```python
from build123d import *

# Parameters (mm, degrees)
CROQUIS1_W              = 77.5
CROQUIS1_H              = 52.5
SALIENTE_EXTRUIR1_DEPTH = 30
VACIADO1_T              = -2
CROQUIS2_R              = 1.75
CORTAR_EXTRUIR1_DEPTH   = 30


with BuildPart() as part:
    # Croquis1 → Saliente-Extruir1 (new body)
    with BuildSketch(Plane(origin=(0, 0, 0), x_dir=(1, 0, 0), z_dir=(0, 1, 0))):
        Rectangle(CROQUIS1_W, CROQUIS1_H)
    extrude(amount=SALIENTE_EXTRUIR1_DEPTH)

    # Vaciado1
    vaciado1_openings = [part.faces().sort_by_distance(p)[0] for p in [
        (0, 30, 0),
    ]]
    offset(amount=VACIADO1_T, openings=vaciado1_openings, kind=Kind.INTERSECTION)

    # Croquis2 → Cortar-Extruir1 (cut, symmetric)
    with BuildSketch(Plane(origin=(0, 2, 0), x_dir=(1, 0, 0), z_dir=(0, 1, 0))):
        with Locations(Location((-36.25, 23.75, 0), (0, 0, 270))):
            Circle(CROQUIS2_R)
        with Locations(Location((36.25, 23.75, 0), (0, 0, 270))):
            Circle(CROQUIS2_R)
        with Locations(Location((36.25, -23.75, 0), (0, 0, 270))):
            Circle(CROQUIS2_R)
        with Locations(Location((-36.25, -23.75, 0), (0, 0, 270))):
            Circle(CROQUIS2_R)
    extrude(amount=CORTAR_EXTRUIR1_DEPTH, both=True, mode=Mode.SUBTRACT)


solid = part.part
```
Design review of the part built by this model. Coordinates are the model's own, in mm. A direction names the side the tool comes from. Coordinates: 2 decimals unless noted, no trailing zeros. Order: outer loops, then holes, each group sorted by start corner. A loop starts at its lowest first (then second) coordinate and runs counter-clockwise, first axis right, second up. Notation, with made-up numbers: M 42,78 L 97,78 A24 ccw 97,114 Z; hole C 12,56 d9. An arc over 180 degrees is marked long. Answer as a JSON object with one key per item and string values. Group by question number.
1) Wall thickness on L1, parallel to Z at x = 36.25, y = 0.5; L2, parallel to X at y = 0.85, z = -23.75; L3, parallel to X at y = 12.5, z = -23.75: over which ranges is each line inside the solid? List them lowest first.
2) Add section A-A, the plane y = 21.5. Write out the cut boundary in (x, z).
3) Mouldability with a two-part tool opening along Z and no side actions: class faces 1 (the flat face through (-1, 15, 26.25)), 2 (the flat face through (-1, 0, 0)), 3 (the flat face through (0, 16, 24.25)) as pulls with the +Z half, pulls with the -Z half, needs draft (parallel to the pull), parting line crosses it, or undercut.
4) Add section B-B, the plane z = 4. Write out the cut boundary in (x, y), then the cut area to 3 significant figures.
5) For pin 1 (1.5 mm diameter, centred on x = -17.5, z = 15.5, fed in from +Y), flat-tipped, find the tip position at first contact; note if it passes through.
6) Add section C-C, the plane x = 16. Write out the cut boundary in (y, z).
7) Tool access review of faces 4 (the flat face through (-1, 2, 0)), 5 (the flat face through (-1, 15, -26.25)): name each direction out of +Z, -Z, +X, -X, +Y, -Y from which nothing blocks a thin tool from reaching the whole face with its end or side.
Computed values:
{
 "1": {"L1": "z = -26.25 to -25.5, -22 to 22, 25.5 to 26.25", "L2": "x = -38.75 to -38, -34.5 to 34.5, 38 to 38.75", "L3": "x = -38.75 to -38, 38 to 38.75"},
 "2": {"outline": "M -38.75,-26.25 L 38.75,-26.25 L 38.75,26.25 L -38.75,26.25 Z; hole M -36.75,-22.07 A1.75 ccw long -34.57,-24.25 L 34.57,-24.25 A1.75 ccw long 36.75,-22.07 L 36.75,22.07 A1.75 ccw long 34.57,24.25 L -34.57,24.25 A1.75 ccw long -36.75,22.07 Z"},
 "3": {"face 1": "pulls with the +Z half", "face 2": "needs draft", "face 3": "undercut"},
 "4": {"outline": "M -38.75,0 L 38.75,0 L 38.75,30 L 36.75,30 L 36.75,2 L -36.75,2 L -36.75,30 L -38.75,30 Z", "area": "267 mm^2"},
 "5": {"pin 1": "stops at y = 2"},
 "6": {"outline": "M 0,-26.25 L 30,-26.25 L 30,-24.25 L 2,-24.25 L 2,24.25 L 30,24.25 L 30,26.25 L 0,26.25 Z"},
 "7": {"face 4": "+Y", "face 5": "-Z, +X, -X, +Y, -Y"}
}
